from build123d import *

# Parameters (mm, degrees)
SKETCH1_W           = 35
SKETCH1_H           = 30
BOSS_EXTRUDE1_DEPTH = 60
SKETCH2_R           = 4
BOSS_EXTRUDE2_DEPTH = 5
SKETCH4_R           = 23.048861143
BOSS_EXTRUDE3_DEPTH = 2
FILLET3_RADIUS      = 15
FILLET3_LENGTH      = 35
FILLET1_R           = 6
SKETCH7_R           = 5
BOSS_EXTRUDE4_DEPTH = 1


with BuildPart() as part:
    # Sketch1 → Boss-Extrude1 (new body)
    with BuildSketch(Plane(origin=(0, 0, 0), x_dir=(1, 0, 0), z_dir=(0, 1, 0))):
        Rectangle(SKETCH1_W, SKETCH1_H)
    extrude(amount=BOSS_EXTRUDE1_DEPTH)

    # Sketch2 → Boss-Extrude2 (add)
    with BuildSketch(Plane(origin=(17.5, 0, 0), x_dir=(0, 0, -1), z_dir=(1, 0, 0))):
        with Locations(Location((0, 45, 0), (0, 0, 180))):
            Circle(SKETCH2_R)
    boss_extrude2 = extrude(amount=BOSS_EXTRUDE2_DEPTH)

    # Mirror1: Boss-Extrude2 across plane
    add(boss_extrude2.mirror(Plane(origin=(0, 0, 0), x_dir=(0, 0, 1), z_dir=(1, 0, 0))))

    # Sketch4 → Boss-Extrude3 (add)
    with BuildSketch(Plane(origin=(0, 0, 0), x_dir=(1, 0, 0), z_dir=(0, 1, 0))):
        with Locations(Location((0, 0, 0), (0, 0, 40.601294645))):
            Circle(SKETCH4_R)
    extrude(amount=BOSS_EXTRUDE3_DEPTH)

    # Fillet3: full round fillet: the end face becomes a half cylinder, R = half its width
    fillet3_face = Plane((0, 60, 0), x_dir=(1, 0, 0), z_dir=(0, 1, 0))  # on the end face: x along it, z out of the body
    fillet3_slab = fillet3_face.offset(-FILLET3_RADIUS / 2) * Box(FILLET3_LENGTH, 2 * FILLET3_RADIUS, FILLET3_RADIUS, mode=Mode.PRIVATE)  # the body's end, R deep
    fillet3_round = Plane((0, 45, 0), x_dir=(0, 1, 0), z_dir=(1, 0, 0)) * Cylinder(FILLET3_RADIUS, FILLET3_LENGTH, mode=Mode.PRIVATE)  # its axis R under the face
    add(fillet3_slab - fillet3_round, mode=Mode.SUBTRACT)

    # Fillet1
    # the kernel refuses this fillet: 6 mm, written as the material it takes off along each edge
    with BuildSketch(Plane(origin=(-17.5, 2, 15), x_dir=(0, 0, -1), z_dir=(0, 1, 0)), Plane(origin=(17.5, 2, 15), x_dir=(-1, 0, 0), z_dir=(0, 1, 0)), Plane(origin=(17.5, 2, -15), x_dir=(0, 0, 1), z_dir=(0, 1, 0))) as fillet1_piece_1:
        with BuildLine():
            CenterArc((FILLET1_R, -FILLET1_R), FILLET1_R, 90, 90)
            Line((0, -FILLET1_R), (0, 0))
            Line((0, 0), (FILLET1_R, 0))
        make_face()
    extrude(amount=43, mode=Mode.SUBTRACT)
    with BuildSketch(Plane(origin=(-17.5, 2, -15), x_dir=(0, 0, 1), z_dir=(0, 1, 0))) as fillet1_piece_2:
        with BuildLine():
            CenterArc((FILLET1_R, FILLET1_R), FILLET1_R, 180, 90)
            Line((0, FILLET1_R), (0, 0))
            Line((0, 0), (FILLET1_R, 0))
        make_face()
    extrude(amount=43, mode=Mode.SUBTRACT)
    with BuildSketch(Plane(origin=(17.5, 45, 0), x_dir=(0, 0, -1), z_dir=(0, -1, 0))) as fillet1_piece_3:
        with BuildLine():
            CenterArc((15 - FILLET1_R, -FILLET1_R), FILLET1_R, 0, 90)
            Line((15, -FILLET1_R), (15, 0))
            Line((15, 0), (15 - FILLET1_R, 0))
        make_face()
    revolve(axis=Axis((17.5, 45, 0), (1, 0, 0)), revolution_arc=180, mode=Mode.SUBTRACT)
    with BuildSketch(Plane(origin=(-17.5, 45, 0), x_dir=(0, 0, 1), z_dir=(0, -1, 0))) as fillet1_piece_4:
        with BuildLine():
            CenterArc((15 - FILLET1_R, -FILLET1_R), FILLET1_R, 0, 90)
            Line((15, -FILLET1_R), (15, 0))
            Line((15, 0), (15 - FILLET1_R, 0))
        make_face()
    revolve(axis=Axis((-17.5, 45, 0), (-1, 0, 0)), revolution_arc=180, mode=Mode.SUBTRACT)

    # Sketch7 → Boss-Extrude4 (add)
    with BuildSketch(Plane.XZ):
        with Locations(Location((0, 0, 0), (0, 0, 270))):
            Circle(SKETCH7_R)
    extrude(amount=BOSS_EXTRUDE4_DEPTH)


solid = part.part
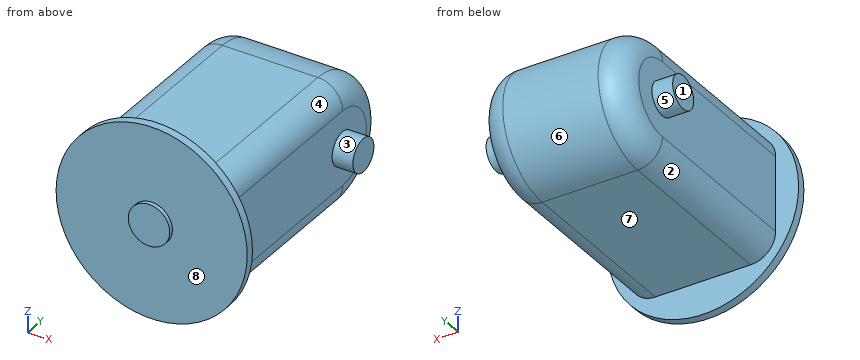
Source: CAD feature listing. Evaluate the final solid. Frame: model axes, mm. Face numbers are marked on the shaded views. A direction names the side the tool comes from. Round coordinates to 2 decimals unless told otherwise and drop trailing zeros. Loops run counter-clockwise (first coordinate to the right, second up) from the corner with the lowest first, then second, coordinate; pieces in that order, holes last. Notation, with made-up numbers: (6, 18.25) - (56, 18.25) arc R15 ccw to (56, 29.25) - close; hole circle Ø10 at (-32, -16). An arc over 180 degrees is marked (long way). Write item = value, one per line. Start each with the question number.
Item 1: Reachability of the marked faces 1, 2, 3 and 4 from +Z, -Z, +X, -X, +Y, -Y: full face, straight path, thin tool, end or side. Return the list, or none.
Item 2: Section query D-D on x = -13. Output: boundary loops of the cut face in (y, z), plus the area to 3 significant figures.
Item 3: Section query B-B on x = 0. Output: boundary loops of the cut face in (y, z), plus the area to 3 significant figures.
Item 4: Section query A-A on y = 13.5. Output: boundary loops of the cut face in (x, z), plus the area to 3 significant figures.
Item 5: Material intervals for line 1 (X direction, y = 8.5, z = 1.5); line 2 (Z direction, x = -6, y = 33); line 3 (Y direction, x = 3, z = 0), sorted ascending.
Item 6: Section query C-C on z = 0. Output: boundary loops of the cut face in (x, y).
Item 7: Mould query, pull axis Y, two halves, no side actions, for the marked faces 5, 6, 7 and 8. Classes: released by +Y, released by -Y, zero draft, split by the parting line, or undercut.
Item 8: First-contact query: pin 1 Ø2 at (y, z) = (36.5, -11) entering from +X; pin 2 Ø4 at (y, z) = (45, 0.5) entering from -X; pin 3 Ø6 at (x, y) = (-7.5, 28.5) entering from +Z. Flat tips, straight axial feed; report the tip coordinate or a pass-through.
Results list:
q1.face_1 = +Z, -Z, -X, +Y
q1.face_2 = -Z, -X, +Y
q1.face_3 = +X
q1.face_4 = +Z, +X, +Y
q2.outline = (0, -19.03) - (2, -19.03) - (2, -14.81) - (45, -14.81) arc R14.81 ccw to (45, 14.81) - (2, 14.81) - (2, 19.03) - (0, 19.03) - close
q2.area = 1,690 mm²
q3.outline = (-1, -5) - (0, -5) - (0, -23.05) - (2, -23.05) - (2, -15) - (45, -15) arc R15 ccw to (45, 15) - (2, 15) - (2, 23.05) - (0, 23.05) - (0, 5) - (-1, 5) - close
q3.area = 1,750 mm²
q4.outline = (-17.5, -9) arc R6 ccw to (-11.5, -15) - (11.5, -15) arc R6 ccw to (17.5, -9) - (17.5, 9) arc R6 ccw to (11.5, 15) - (-11.5, 15) arc R6 ccw to (-17.5, 9) - close
q4.area = 1,020 mm²
q5.line_1 = -17.5 to 17.5
q5.line_2 = -15 to 15
q5.line_3 = -1 to 60
q6.outline = (-23.05, 0) - (-5, 0) - (-5, -1) - (5, -1) - (5, 0) - (23.05, 0) - (23.05, 2) - (17.5, 2) - (17.5, 41) - (22.5, 41) - (22.5, 49) - (17.5, 49) - (17.5, 54) arc R6 ccw to (11.5, 60) - (-11.5, 60) arc R6 ccw to (-17.5, 54) - (-17.5, 49) - (-22.5, 49) - (-22.5, 41) - (-17.5, 41) - (-17.5, 2) - (-23.05, 2) - close
q7.face_5 = undercut
q7.face_6 = released by +Y
q7.face_7 = zero draft
q7.face_8 = released by -Y
q8.pin_1 = 17.42
q8.pin_2 = -22.5
q8.pin_3 = 15
